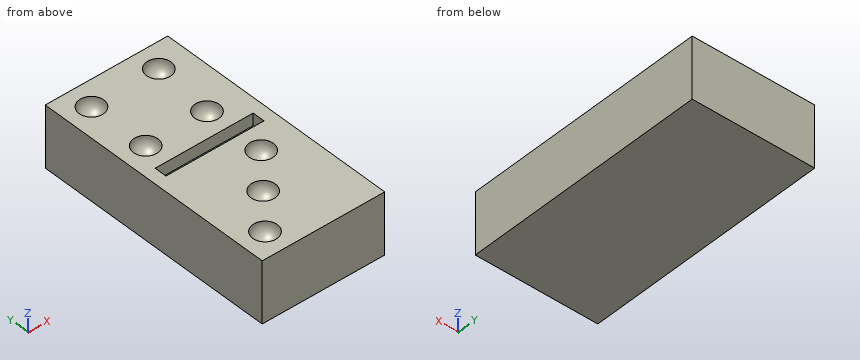
from build123d import *

# Parameters (mm, degrees)
SPHERE_ANGLE    = 180
SPHERE002_ANGLE = 180
SPHERE001_ANGLE = 180
SPHERE003_ANGLE = 180
SPHERE004_ANGLE = 180
SPHERE005_ANGLE = 180
SPHERE006_ANGLE = 180
SPHERE007_ANGLE = 180
BOX001_W        = 8
BOX001_H        = 1
BOX001_DEPTH    = 1
BOX_W           = 10
BOX_H           = 20
BOX_DEPTH       = 5


with BuildPart() as esfera:
    # Sphere → Sphere (revolve)
    with BuildSketch(Plane(origin=(2, 2, 5), x_dir=(1, 0, 0), z_dir=(0, 0, 1))):
        with BuildLine():
            ThreePointArc((0, -1), (1, 0), (0, 1))
            Line((0, 1), (0, -1))
        make_face()
    revolve(axis=Axis((2, 2, 5), (0, 1, 0)), revolution_arc=SPHERE_ANGLE)


with BuildPart() as esfera002:
    # Sphere002 → Sphere002 (revolve)
    with BuildSketch(Plane(origin=(7, 8, 5), x_dir=(1, 0, 0), z_dir=(0, 0, 1))):
        with BuildLine():
            ThreePointArc((0, -1), (1, 0), (0, 1))
            Line((0, 1), (0, -1))
        make_face()
    revolve(axis=Axis((7, 8, 5), (0, 1, 0)), revolution_arc=SPHERE002_ANGLE)


with BuildPart() as esfera001:
    # Sphere001 → Sphere001 (revolve)
    with BuildSketch(Plane(origin=(4.5, 5, 5), x_dir=(1, 0, 0), z_dir=(0, 0, 1))):
        with BuildLine():
            ThreePointArc((0, -1), (1, 0), (0, 1))
            Line((0, 1), (0, -1))
        make_face()
    revolve(axis=Axis((4.5, 5, 5), (0, 1, 0)), revolution_arc=SPHERE001_ANGLE)


with BuildPart() as esfera003:
    # Sphere003 → Sphere003 (revolve)
    with BuildSketch(Plane(origin=(4.5, 5, 5), x_dir=(1, 0, 0), z_dir=(0, 0, 1))):
        with BuildLine():
            ThreePointArc((0, -1), (1, 0), (0, 1))
            Line((0, 1), (0, -1))
        make_face()
    revolve(axis=Axis((4.5, 5, 5), (0, 1, 0)), revolution_arc=SPHERE003_ANGLE)


with BuildPart() as esfera004:
    # Sphere004 → Sphere004 (revolve)
    with BuildSketch(Plane(origin=(7.5, 18, 5), x_dir=(1, 0, 0), z_dir=(0, 0, 1))):
        with BuildLine():
            ThreePointArc((0, -1), (1, 0), (0, 1))
            Line((0, 1), (0, -1))
        make_face()
    revolve(axis=Axis((7.5, 18, 5), (0, 1, 0)), revolution_arc=SPHERE004_ANGLE)


with BuildPart() as esfera005:
    # Sphere005 → Sphere005 (revolve)
    with BuildSketch(Plane(origin=(2, 18, 5), x_dir=(1, 0, 0), z_dir=(0, 0, 1))):
        with BuildLine():
            ThreePointArc((0, -1), (1, 0), (0, 1))
            Line((0, 1), (0, -1))
        make_face()
    revolve(axis=Axis((2, 18, 5), (0, 1, 0)), revolution_arc=SPHERE005_ANGLE)


with BuildPart() as esfera006:
    # Sphere006 → Sphere006 (revolve)
    with BuildSketch(Plane(origin=(2, 13, 5), x_dir=(1, 0, 0), z_dir=(0, 0, 1))):
        with BuildLine():
            ThreePointArc((0, -1), (1, 0), (0, 1))
            Line((0, 1), (0, -1))
        make_face()
    revolve(axis=Axis((2, 13, 5), (0, 1, 0)), revolution_arc=SPHERE006_ANGLE)


with BuildPart() as esfera007:
    # Sphere007 → Sphere007 (revolve)
    with BuildSketch(Plane(origin=(7, 13, 5), x_dir=(1, 0, 0), z_dir=(0, 0, 1))):
        with BuildLine():
            ThreePointArc((0, -1), (1, 0), (0, 1))
            Line((0, 1), (0, -1))
        make_face()
    revolve(axis=Axis((7, 13, 5), (0, 1, 0)), revolution_arc=SPHERE007_ANGLE)


with BuildPart() as fusion:
    # Box001 → Box001 (new body)
    with BuildSketch(Plane(origin=(1, 10, 4), x_dir=(1, 0, 0), z_dir=(0, 0, 1))):
        with Locations((4, 0.5)):
            Rectangle(BOX001_W, BOX001_H)
    extrude(amount=BOX001_DEPTH)

    # Fusion: union Esfera, Esfera002, Esfera001, Esfera003, Esfera004, Esfera005, Esfera006, Esfera007
    add(esfera.part)
    add(esfera002.part)
    add(esfera001.part)
    add(esfera003.part)
    add(esfera004.part)
    add(esfera005.part)
    add(esfera006.part)
    add(esfera007.part)


with BuildPart() as cut:
    # Box → Box (new body)
    with BuildSketch(Plane.XY):
        with Locations((5, 10)):
            Rectangle(BOX_W, BOX_H)
    extrude(amount=BOX_DEPTH)

    # Cut: cut Fusion
    add(fusion.part, mode=Mode.SUBTRACT)


solid = cut.part
CAD build for the part. Positions are in the model's coordinates, mm. Round coordinates to 2 decimals unless told otherwise and drop trailing zeros. Write each loop counter-clockwise with the first axis right and the second up, starting at its lowest first coordinate (ties: lowest second). Pieces come first, ordered by that corner, then holes. Notation, with made-up numbers: (37.5, 31) -> (42.5, 31) arc R18 ccw to (42.5, 43) -> close; hole circle Ø3 at (26.5, 71.25). An arc over 180 degrees is marked (long way). Answer as a JSON object with one key per item and string values.
(1) Band-saw the part on D-D, the plane x = 2.75. List the corners of the cut face in (y, z).
Reported:
{"outline": "(0, 0) -> (20, 0) -> (20, 5) -> (18.66, 5) arc R0.66 cw to (17.34, 5) -> (13.66, 5) arc R0.66 cw to (12.34, 5) -> (11, 5) -> (11, 4) -> (10, 4) -> (10, 5) -> (2.66, 5) arc R0.66 cw to (1.34, 5) -> (0, 5) -> close"}
(2) Probe probe 1 along Y at (x, z) = (6, 4.5); probe 2 along Y at (x, z) = (7, 4.45); probe 3 along Y at (x, z) = (2, 4.6). List the from-to ranges inside material, lowest first. Write a range as [from, to].
Reported:
{"probe 1": "y = [0, 10], [11, 20]", "probe 2": "y = [0, 7.16], [8.84, 10], [11, 12.16], [13.84, 17.33], [18.67, 20]", "probe 3": "y = [0, 1.08], [2.92, 10], [11, 12.08], [13.92, 17.08], [18.92, 20]"}
(3) Band-saw the part on B-B, the plane x = 1.75. List the corners of the cut face in (y, z), then the cut area to 3 significant figures.
Reported:
{"outline": "(0, 0) -> (20, 0) -> (20, 5) -> (18.97, 5) arc R0.97 cw to (17.03, 5) -> (13.97, 5) arc R0.97 cw to (12.03, 5) -> (11, 5) -> (11, 4) -> (10, 4) -> (10, 5) -> (2.97, 5) arc R0.97 cw to (1.03, 5) -> (0, 5) -> close", "area": "94.6 mm^2"}
(4) Band-saw the part on A-A, the plane z = 4.35. Count the separate pieces of the cut face and the enclosed holes in it, then the cut area to 3 significant figures.
Reported:
{"separate pieces": "1", "enclosed holes": "8", "area": "179 mm^2"}
(5) Band-saw the part on C-C, the plane y = 2. List the corners of the cut face in (x, z), then the cut area to 3 significant figures.
Reported:
{"outline": "(0, 0) -> (10, 0) -> (10, 5) -> (3, 5) arc R1 cw to (1, 5) -> (0, 5) -> close", "area": "48.4 mm^2"}
